Geometry check sheet. Reference: drawing and pictorial views, mm from the part's lowest x, y, z. A direction names the side the tool comes from. Give positions to 0.01 mm unless a question says otherwise; leave off trailing zeros. Write each loop counter-clockwise with the first axis right and the second up, starting at its lowest first coordinate (ties: lowest second). Pieces come first, ordered by that corner, then holes. Notation, with made-up numbers: M 62.25,71.5 L 82.25,71.5 A24 cw 82.25,85.5 Z; hole C 52.5,29 d8. An arc over 180 degrees is marked long. Write each question's results on one line, items separated by ' | '. Start each with the question number.
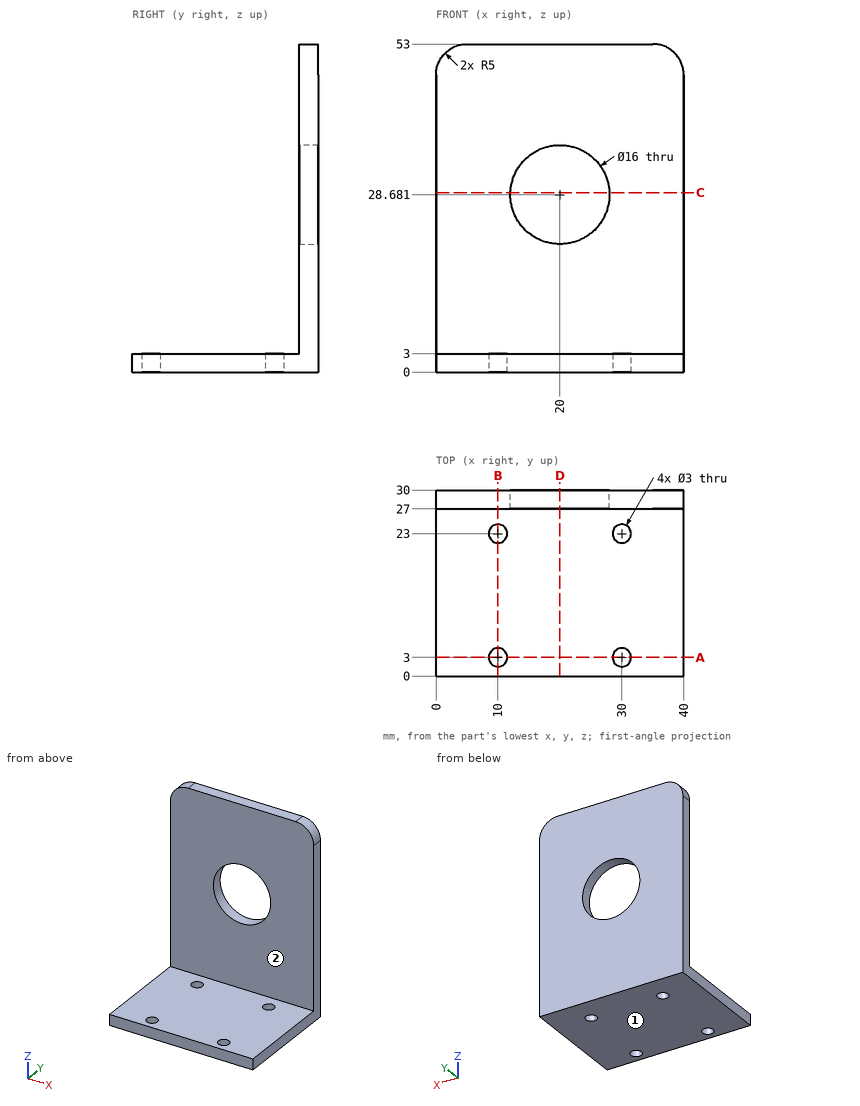
Q1. Section check C-C on z = 29. Record the boundary of the cut face in (x, y), plus the area to 3 significant figures.
Q2. Section check A-A on y = 3. Record the boundary of the cut face in (x, z), plus the area to 3 significant figures.
Q3. Section check D-D on x = 20. Record the boundary of the cut face in (y, z), plus the area to 3 significant figures.
Q4. Tool access check on the marked faces 1 and 2. Record the directions out of +Z, -Z, +X, -X, +Y, -Y that give a thin tool (end or side, any length) a straight path to the whole face; none if there is none.
Q5. Section check B-B on x = 10. Record the boundary of the cut face in (y, z), plus the area to 3 significant figures.
Q6. Depth check by flat-ended pin: pin 1 Ø4 at (x, y) = (10, 23) entering from +Z; pin 2 Ø1 at (x, z) = (10.5, 38.5) entering from -Y; pin 3 Ø2.5 at (x, y) = (30, 3) entering from +Z. Enter the tip coordinate at first touch or a pass-through.
Q7. Scan lines: L1, parallel to Y at x = 30, z = 0.95; L2, parallel to Y at x = 30, z = 41.5; L3, parallel to Z at x = 12.5, y = 15.25. Record each from-to range of solid material in increasing order.
Check result:
1) outline: M 0,27 L 12.01,27 L 12.01,30 L 0,30 Z; M 27.99,27 L 40,27 L 40,30 L 27.99,30 Z | area: 72.0 mm^2
2) outline: M 0,0 L 8.5,0 L 8.5,3 L 0,3 Z; M 11.5,0 L 28.5,0 L 28.5,3 L 11.5,3 Z; M 31.5,0 L 40,0 L 40,3 L 31.5,3 Z | area: 102 mm^2
3) outline: M 0,0 L 30,0 L 30,20.68 L 27,20.68 L 27,3 L 0,3 Z; M 27,36.68 L 30,36.68 L 30,53 L 27,53 Z | area: 192 mm^2
4) face 1: -Z, +X, -X, +Y, -Y | face 2: +Z, +X, -X, -Y
5) outline: M 0,0 L 1.5,0 L 1.5,3 L 0,3 Z; M 4.5,0 L 21.5,0 L 21.5,3 L 4.5,3 Z; M 24.5,0 L 30,0 L 30,53 L 27,53 L 27,3 L 24.5,3 Z | area: 222 mm^2
6) pin 1: z = 3 | pin 2: y = 27 | pin 3: through
7) L1: 0 to 1.5, 4.5 to 21.5, 24.5 to 30 | L2: 27 to 30 | L3: 0 to 3
